```python
from build123d import *

# Parameters (mm, degrees)
ESQUISSE2_W                  = 38
ESQUISSE2_H                  = 32
BOSS_EXTRU_1_DEPTH           = 3
ESQUISSE3_R                  = 2
ESQUISSE3_R_2                = 2.25
ENL_V_MAT_EXTRU_1_DEPTH      = 1
ENL_V_MAT_EXTRU_1_DEPTH_BACK = 4
ESQUISSE4_R                  = 2.5
ENL_V_MAT_EXTRU_2_DEPTH      = 0.4
ESQUISSE5_W                  = 8
ESQUISSE5_H                  = 6
ENL_V_MAT_EXTRU_3_DEPTH      = 1
ENL_V_MAT_EXTRU_3_DEPTH_BACK = 4
CONG_1_R                     = 2


with BuildPart() as part:
    # Esquisse2 → Boss.-Extru.1 (new body)
    with BuildSketch(Plane.XY):
        with Locations((19, 16)):
            Rectangle(ESQUISSE2_W, ESQUISSE2_H)
    extrude(amount=BOSS_EXTRU_1_DEPTH)

    # Esquisse3 → Enlèv. mat.-Extru.1 (cut, two sides)
    with BuildSketch(Plane.XY.offset(3)) as enl_v_mat_extru_1_sk:
        with Locations((19, 28)):
            Circle(ESQUISSE3_R)
        with Locations((13, 28)):
            Circle(ESQUISSE3_R)
        with Locations((25, 28)):
            Circle(ESQUISSE3_R)
        with Locations((25, 4)):
            Circle(ESQUISSE3_R)
        with Locations((13, 4)):
            Circle(ESQUISSE3_R)
        with Locations((19, 4)):
            Circle(ESQUISSE3_R)
        with Locations((4, 22)):
            Circle(ESQUISSE3_R_2)
        with Locations((4, 10)):
            Circle(ESQUISSE3_R_2)
        with Locations((34, 10)):
            Circle(ESQUISSE3_R_2)
        with Locations((34, 22)):
            Circle(ESQUISSE3_R_2)
    extrude(amount=ENL_V_MAT_EXTRU_1_DEPTH, mode=Mode.SUBTRACT)
    extrude(enl_v_mat_extru_1_sk.sketch, amount=-ENL_V_MAT_EXTRU_1_DEPTH_BACK, mode=Mode.SUBTRACT)

    # Esquisse4 → Enlèv. mat.-Extru.2 (cut)
    with BuildSketch(Plane.XY.offset(3)):
        with Locations((13, 4)):
            Circle(ESQUISSE4_R)
        with Locations((19, 4)):
            Circle(ESQUISSE4_R)
        with Locations((25, 4)):
            Circle(ESQUISSE4_R)
        with Locations((25, 28)):
            Circle(ESQUISSE4_R)
        with Locations((19, 28)):
            Circle(ESQUISSE4_R)
        with Locations((13, 28)):
            Circle(ESQUISSE4_R)
    extrude(amount=-ENL_V_MAT_EXTRU_2_DEPTH, mode=Mode.SUBTRACT)

    # Esquisse5 → Enlèv. mat.-Extru.3 (cut, two sides)
    with BuildSketch(Plane.XY.offset(3)) as enl_v_mat_extru_3_sk:
        with Locations((4, 29)):
            Rectangle(ESQUISSE5_W, ESQUISSE5_H)
        with Locations((34, 29)):
            Rectangle(ESQUISSE5_W, ESQUISSE5_H)
        with Locations((34, 3)):
            Rectangle(ESQUISSE5_W, ESQUISSE5_H)
        with Locations((4, 3)):
            Rectangle(ESQUISSE5_W, ESQUISSE5_H)
    extrude(amount=ENL_V_MAT_EXTRU_3_DEPTH, mode=Mode.SUBTRACT)
    extrude(enl_v_mat_extru_3_sk.sketch, amount=-ENL_V_MAT_EXTRU_3_DEPTH_BACK, mode=Mode.SUBTRACT)

    # Congé1
    cong_1_edges = [part.edges().sort_by_distance(p)[0] for p in [
        (0, 26, 1.5),
        (8, 32, 1.5),
        (8, 26, 1.5),
        (30, 32, 1.5),
        (38, 26, 1.5),
        (30, 26, 1.5),
        (38, 6, 1.5),
        (30, 0, 1.5),
        (30, 6, 1.5),
        (8, 0, 1.5),
        (0, 6, 1.5),
        (8, 6, 1.5),
    ]]
    fillet(cong_1_edges, radius=CONG_1_R)


solid = part.part
```
The model under review builds one solid part; all positions refer to its coordinate system, in mm. A direction names the side the tool comes from. Round coordinates to 2 decimals unless told otherwise and drop trailing zeros. Write each loop counter-clockwise with the first axis right and the second up, starting at its lowest first coordinate (ties: lowest second). Pieces come first, ordered by that corner, then holes. Notation, with made-up numbers: (-27, -11.5) -> (5, -11.5) arc R22 ccw to (5, 0.5) -> close; hole circle Ø2 at (-1, 77.25). An arc over 180 degrees is marked (long way). Use CSV: the item, a comma, the result in double quotes.
Q1. Mouldability with a two-part tool opening along Y and no side actions: class faces 1 (the cylindrical face through (0.57, 25.4, 1.48)), 2 (the cylindrical face through (29.43, 0.6, 1.48)), 3 (the cylindrical face through (11.4, 2.8, 1.3)) as released by +Y, released by -Y, zero draft, split by the parting line, or undercut.
Checks:
face 1,"released by +Y"
face 2,"released by -Y"
face 3,"undercut"
Q2. Consider section D-D (x = 35.5). Give the boundary of the cut face in (y, z), then the cut area to 3 significant figures.
Checks:
outline,"(6, 0) -> (8.32, 0) -> (8.32, 3) -> (6, 3) -> close; (11.68, 0) -> (20.32, 0) -> (20.32, 3) -> (11.68, 3) -> close; (23.68, 0) -> (26, 0) -> (26, 3) -> (23.68, 3) -> close"
area,"39.9 mm²"
Q3. For pin 1 Ø8 at (x, y) = (5, 16.5) entering from -Z; pin 2 Ø3 at (x, y) = (13, 4) entering from -Z; pin 3 Ø1.5 at (x, z) = (29.5, 2) entering from -Y; pin 4 Ø1.6 at (y, z) = (28.5, 1) entering from +X, all flat-tipped, find the tip position at first contact; note any pin that passes through.
Checks:
pin 1,"z = 0"
pin 2,"through"
pin 3,"y = 0.15"
pin 4,"x = 30.02"
Q4. Consider section B-B (z = 0.5). State how many separate pieces and enclosed holes the cut face has, then the cut area to 3 significant figures.
Checks:
separate pieces,"1"
enclosed holes,"10"
area,"882 mm²"
Q5. To check wall thickness, follow probe 1 along Y at (x, z) = (4, 2.3); probe 2 along Y at (x, z) = (13, 1.05); probe 3 along X at (y, z) = (20, 2.3). State the ranges of each line that lie inside material, in increasing order. Write a range as [from, to].
Checks:
probe 1,"[6, 7.75], [12.25, 19.75], [24.25, 26]"
probe 2,"[0, 2], [6, 26], [30, 32]"
probe 3,"[0, 2.97], [5.03, 32.97], [35.03, 38]"
Q6. Consider section A-A (x = 13). Give the boundary of the cut face in (y, z), then the cut area to 3 significant figures.
Checks:
outline,"(0, 0) -> (2, 0) -> (2, 2.6) -> (1.5, 2.6) -> (1.5, 3) -> (0, 3) -> close; (6, 0) -> (26, 0) -> (26, 2.6) -> (25.5, 2.6) -> (25.5, 3) -> (6.5, 3) -> (6.5, 2.6) -> (6, 2.6) -> close; (30, 0) -> (32, 0) -> (32, 3) -> (30.5, 3) -> (30.5, 2.6) -> (30, 2.6) -> close"
area,"71.2 mm²"
Q7. For faces 4 (the flat face through (30, 3, 2)), 5 (the flat face through (12, 6, 2.6)), 6 (the flat face through (19, 0, 1)), 7 (the flat face through (19, 16, 3)), 8 (the flat face through (8, 3, 2)), list the 3-axis set-ups (+Z, -Z, +X, -X, +Y, -Y) from which the entire face can be reached by the end or side of a thin tool; tool diameter is ignored.
Checks:
face 4,"+Z, -Z, +X, -Y"
face 5,"+Z"
face 6,"+Z, -Z, +X, -X, -Y"
face 7,"+Z, +X, -X, +Y, -Y"
face 8,"+Z, -Z, -X, -Y"
Q8. Consider section C-C (y = 22). Give the boundary of the cut face in (x, z).
Checks:
outline,"(0, 0) -> (1.75, 0) -> (1.75, 3) -> (0, 3) -> close; (6.25, 0) -> (31.75, 0) -> (31.75, 3) -> (6.25, 3) -> close; (36.25, 0) -> (38, 0) -> (38, 3) -> (36.25, 3) -> close"
